Input: part model. Units: mm. Frame: model coordinates. A direction names the side the tool comes from. Coordinates: 2 decimals unless noted, no trailing zeros. Write each loop counter-clockwise with the first axis right and the second up, starting at its lowest first coordinate (ties: lowest second). Pieces come first, ordered by that corner, then holes. Notation, with made-up numbers: (-39, 80.25) - (-25, 80.25) arc R17 ccw to (-25, 93.25) - close; hole circle Ø2 at (86.5, -19). An arc over 180 degrees is marked (long way). Use a Markdown table: item, result. Add a question column.
Q1. Set-up query: faces 1 (the face through (6, 0, 2)), 2 (the face through (-20.641, -0.143, 3.033)). Return all of +Z, -Z, +X, -X, +Y, -Y with unobstructed straight access to the full face (end or side cutting, diameter ignored); none if empty.
Q2. Section query A-A (y = 0). Return the cut outline in (x, z) (1 decimal), then the cut area to 3 significant figures.
Q3. Section query D-D (x = -12). Return the cut outline in (y, z) (3 decimals).
Q4. Pin query (flat end, axial travel): P1, Ø12, axis at x = 14, y = 2.5, coming from the -Z side (3 decimals); P2, Ø3, axis at x = -7.5, z = 0.5, coming from the -Y side; P3, Ø3, axis at x = 0, z = -1, coming from the +Y side. Return the tip coordinate at first contact, or that it passes through.
Q5. Section query B-B (x = 12). Return the cut outline in (y, z) (3 decimals), then the cut area to 3 significant figures.
Q6. Material intervals for probe 1 along Y at (x, z) = (14, 1.5); probe 2 along Y at (x, z) = (-14, -1.25); probe 3 along X at (y, z) = (2.5, 1.75), sorted ascending. Write a range as from..to.
Q7. Section query C-C (z = 0.75). Give the number of separate pieces and of enclosed holes in the cut face, then the cut area to 3 significant figures.
Q8. Mould query, pull axis X, two halves, no side actions, for faces 3 (the face through (0.27, 7.65, 0.21)), 4 (the face through (-2.081, 10.384, -0.037)), 5 (the face through (0, 5, 3.175)). Classes: released by +X, released by -X, zero draft, split by the parting line, or undercut.
Autodesk Inventor part; units mm, degrees
ref_plane "YZ Plane" through (0, 0, 0) normal (1, 0, 0) x (0, 1, 0)
ref_plane "XZ Plane" through (0, 0, 0) normal (0, 1, 0) x (-1, 0, 0)
ref_plane "XY Plane" through (0, 0, 0) normal (0, 0, 1) x (1, 0, 0)
sketch "Sketch1" plane through (0, 0, 0) normal (0, 0, 1) x (1, 0, 0)
  line L0 (-14, 0) -> (14, 0) construction
  line L1 (-14.25, 6.9955) -> (13.7143, 7.9949)
  line L2 (13.7143, -7.9949) -> (-14.25, -6.9955)
  arc A0 (-14.25, 6.9955) -> (-14.25, -6.9955) centre (-14, 0) ccw
  arc A1 (13.7143, -7.9949) -> (13.7143, 7.9949) centre (14, 0) ccw
  line L3 (-7.032, 7.2535) -> (3.1108, 13.6663)
  line L4 (3.1108, 13.6663) -> (6.8515, 7.7496)
  line L5 (4.9811, 10.708) -> (-0.0902, 7.5016) construction
  point P0 (0, 0)
  point P1 (0, 0)
  dimension "d0" = 8
  dimension "d1" = 7
  dimension "d2" = 28
  dimension "d3" = 12
  dimension "d4" = 7
  dimension "d5" = 3.5
  dimension "d6" = 14
extrude "Extrusion1" add sketch "Sketch1" along normal mid plane 6.35
hole "Hole1" at (14, 0, 3.175) direction (0, 0, -1) diameter 7.9375 end through all
hole "Hole2" at (-14, 0, 3.175) direction (0, 0, -1) diameter 9 end through all
sketch "Sketch2" plane through (3.1108, 13.6663, 3.175) normal (0.8452325, 0.5343988, 0) x (0, 0, -1)
  point P0 (3.175, -9.8888)
sketch "Sketch3" plane through (3.1108, 13.6663, 3.175) normal (0.8452325, 0.5343988, 0) x (0, 0, -1)
  line L0 (0, -7) -> (0, 0) construction
  line L1 (0, -3.5) -> (6.35, -3.5) construction
  line L2 (6.35, 0) -> (6.35, -7) construction
  line L3 (6.35, 0) -> (0, 0) construction
  line L4 (3.175, 0) -> (3.175, -7) construction
  line L5 (6.35, -7) -> (0, -7) construction
  point P0 (3.175, -9.8888)
  point P1 (3.175, -3.5)
hole "Hole3" at (4.9811, 10.708, 0) direction (-0.8452325, -0.5343988, 0) diameter 2.487 depth 5 tip angle 118
sketch "Sketch4" plane through (0, 0, 3.175) normal (0, 0, 1) x (1, 0, 0)
  circle A0 centre (-14, 0) radius 4.5
  circle A1 centre (14, 0) radius 3.9687
  line L0 (6.8515, 7.7496) -> (3.1108, 13.6663)
  line L1 (3.1108, 13.6663) -> (-7.032, 7.2535)
  line L2 (-7.032, 7.2535) -> (-14.25, 6.9955)
  arc A2 (-14.25, 6.9955) -> (-14.25, -6.9955) centre (-14, 0) ccw
  line L3 (-14.25, -6.9955) -> (13.7143, -7.9949)
  arc A3 (13.7143, -7.9949) -> (13.7143, 7.9949) centre (14, 0) ccw
  line L4 (13.7143, 7.9949) -> (6.8515, 7.7496)
  line L5 (7.5804, -4.7738) -> (-8.402, -4.2026)
  arc A4 (-8.402, -4.2026) -> (-8.402, 4.2026) centre (-14, 0) ccw
  arc A5 (7.5804, 4.7738) -> (7.5804, -4.7738) centre (14, 0) ccw
  line L6 (-8.402, 4.2026) -> (7.5804, 4.7738)
  point P0 (0, 0)
  dimension "d35" = 3
  dimension "d36" = 3
extrude "Extrusion2" cut sketch "Sketch4" against normal blind 3.175 contours L5 A4 L6 A5
fillet "Fillet1" radius 1.5875 8 edges at (6, 0, 0) (7.5804, 4.7738, 1.5875) (-0.4108, 4.4882, 0) (-8.402, 4.2026, 1.5875) (-7, 0, 0) (-0.4108, -4.4882, 0) (7.5804, -4.7738, 1.5875) (-8.402, -4.2026, 1.5875)
chamfer "Chamfer1" distance 0.5 angle 45 14 edges at (-1.9606, 10.4599, -3.175) (-1.9606, 10.4599, 3.175) (-10.641, 7.1245, -3.175) (-21, 0, -3.175) (-0.2679, -7.4952, -3.175) (22, 0, -3.175) (10.2829, 7.8723, -3.175) (-10.641, 7.1245, 3.175) (-21, 0, 3.175) (-0.2679, -7.4952, 3.175) (22, 0, 3.175) (10.2829, 7.8723, 3.175) (4.9811, 10.708, -3.175) (4.9811, 10.708, 3.175)
fillet "Fillet2" radius 1 1 edges at (3.1108, 13.6663, 0)
fillet "Fillet3" radius 3.175 1 edges at (-7.032, 7.2535, 0)
properties part number "INVENTOR WORKSHOP"
Values follow:
| question | item | result |
|---|---|---|
| 1 | face 1 | +Z |
| 1 | face 2 | +Z, -X |
| 2 | outline | (-21, -2.7) - (-20.5, -3.2) - (-18.5, -3.2) - (-18.5, 3.2) - (-20.5, 3.2) - (-21, 2.7) - close; (-9.5, -3.2) - (10, -3.2) - (10, 3.2) - (6, 3.2) - (6, 1.6) arc R1.6 cw to (4.4, 0) - (-5.4, 0) arc R1.6 cw to (-7, 1.6) - (-7, 3.2) - (-9.5, 3.2) - close; (18, -3.2) - (21.5, -3.2) - (22, -2.7) - (22, 2.7) - (21.5, 3.2) - (18, 3.2) - close |
| 2 | area | 125 mm2 |
| 3 | outline | (-7.076, -2.675) - (-6.576, -3.175) - (-4.031, -3.175) - (-4.031, 3.175) - (-6.576, 3.175) - (-7.076, 2.675) - close; (4.031, -3.175) - (6.576, -3.175) - (7.076, -2.675) - (7.076, 2.675) - (6.576, 3.175) - (4.031, 3.175) - close |
| 4 | P1 | z = -3.175 |
| 4 | P2 | y = -7.29 |
| 4 | P3 | y = 12.65 |
| 5 | outline | (-7.934, -2.675) - (-7.433, -3.175) - (-3.428, -3.175) - (-3.428, 3.175) - (-7.433, 3.175) - (-7.934, 2.675) - close; (3.428, -3.175) - (7.433, -3.175) - (7.934, -2.675) - (7.934, 2.675) - (7.433, 3.175) - (3.428, 3.175) - close |
| 5 | area | 56.7 mm2 |
| 6 | probe 1 | -8..-3.97, 3.97..8 |
| 6 | probe 2 | -7..-4.5, 4.5..7 |
| 6 | probe 3 | -20.54..-17.74, -10.26..-7.42, 6.4..10.92, 17.08..21.6 |
| 7 | separate pieces | 1 |
| 7 | enclosed holes | 3 |
| 7 | area | 407 mm2 |
| 8 | face 3 | undercut |
| 8 | face 4 | released by -X |
| 8 | face 5 | zero draft |
